Source: CAD feature listing. Evaluate the final solid. Frame: model axes, mm. A direction names the side the tool comes from. Coordinates: 2 decimals unless noted, no trailing zeros. Loops run counter-clockwise (first coordinate to the right, second up) from the corner with the lowest first, then second, coordinate; pieces in that order, holes last. Notation, with made-up numbers: M 34.25,42 L 92.25,42 A16 ccw 92.25,46 Z; hole C 42,62.25 d7. An arc over 180 degrees is marked long. Write each question's results on one line, items separated by ' | '. Start each with the question number.
from build123d import *

# Parameters (mm, degrees)
CHAMFER1_SIZE           = 0.4
EXTRUDE1_START          = -3.25
SKETCH2_R               = 11.925743973
EXTRUDE1_DEPTH          = 3.25
EXTRUDE2_START          = -8.8
SKETCH3_R               = 13.491172398
EXTRUDE2_DEPTH          = 8.8
SKETCH4_W               = 1
SKETCH4_H               = 1.144643989
EXTRUDE3_DEPTH          = 9.5
CUT_EXTRUDE1_DEPTH      = 48.023611133
CUT_EXTRUDE1_DEPTH_BACK = 48.023611133
SKETCH5_R               = 0.520703833
SKETCH6_R               = 1.016043674
CUT_EXTRUDE2_DEPTH      = 0.5
CUT_EXTRUDE3_START      = -0.5
SKETCH7_R               = 1.016043674
CUT_EXTRUDE3_DEPTH      = 0.5


with BuildPart() as part:
    # Sketch1 → Revolve1 (revolve)
    with BuildSketch(Plane.XY, mode=Mode.PRIVATE) as revolve1_sk:
        Polygon((0, 0), (0, 5), (1.5, 5), (1.5, 6.275), (11, 6.275), (11, 8.75), (10.5, 8.75), (10.5, 11), (19.3, 11), (19.3, 6.5), (20.3, 6.5), (20.3, 8.4), (24.65, 8.4), (24.65, 10.75), (27.9, 10.75), (27.9, 3.82), (40, 3.82), (40, 2.3), (38, 2.3), (38, 1.6), (12, 1.6), (12, 0), align=None)
    revolve(revolve1_sk.sketch.rotate(Axis((0, 0, 0), (1, 0, 0)), 90), axis=Axis((0, 0, 0), (1, 0, 0)))

    # Chamfer1
    chamfer1_edges = [part.edges().sort_by_distance(p)[0] for p in [
        (40, 0, -3.82),
    ]]
    chamfer(chamfer1_edges, length=CHAMFER1_SIZE)

    # Sketch2 → Extrude1 (cut)
    with BuildSketch(Plane(origin=(27.9, 0, 0), x_dir=(0, 0, -1), z_dir=(1, 0, 0)).offset(EXTRUDE1_START)):
        Circle(SKETCH2_R)
        Polygon((0, 10.75), (-9.309773091, 5.375), (-9.309773091, -5.375), (0, -10.75), (9.309773091, -5.375), (9.309773091, 5.375), align=None, mode=Mode.SUBTRACT)
    extrude(amount=EXTRUDE1_DEPTH, mode=Mode.SUBTRACT)

    # Sketch3 → Extrude2 (cut)
    with BuildSketch(Plane(origin=(19.3, 0, 0), x_dir=(0, 0, -1), z_dir=(1, 0, 0)).offset(EXTRUDE2_START)):
        Circle(SKETCH3_R)
        Polygon((-5.5, 9.526279442), (-11, 0), (-5.5, -9.526279442), (5.5, -9.526279442), (11, 0), (5.5, 9.526279442), align=None, mode=Mode.SUBTRACT)
    extrude(amount=EXTRUDE2_DEPTH, mode=Mode.SUBTRACT)

    # Sketch4 → Extrude3 (cut)
    with BuildSketch(Plane.ZY.offset(-1.5)):
        with Locations((0, 6.063519509)):
            Rectangle(SKETCH4_W, SKETCH4_H)
    extrude(amount=-EXTRUDE3_DEPTH, mode=Mode.SUBTRACT)

    # Sketch5 → Cut-Extrude1 (cut, two sides: drawn at the far end of the back side and taken through both)
    with BuildSketch(Plane(origin=(0, -4.763139721, 8.25), x_dir=(1, 0, 0), z_dir=(0, -0.5000000000000002, 0.8660254037844386)).offset(-CUT_EXTRUDE1_DEPTH_BACK)):
        with Locations(Location((18.145997854, 9.8, 0), (0, 0, 270))):
            Circle(SKETCH5_R)
    extrude(amount=CUT_EXTRUDE1_DEPTH + CUT_EXTRUDE1_DEPTH_BACK, mode=Mode.SUBTRACT)

    # Sketch6 → Cut-Extrude2 (cut)
    with BuildSketch(Plane(origin=(0, -4.763139721, 8.25), x_dir=(1, 0, 0), z_dir=(0, -0.5000000000000002, 0.8660254037844386))):
        with Locations(Location((16.808700708, 2.994097786, 0), (0, 0, 270))):
            Circle(SKETCH6_R)
    extrude(amount=-CUT_EXTRUDE2_DEPTH, mode=Mode.SUBTRACT)

    # Sketch7 → Cut-Extrude3 (cut)
    with BuildSketch(Plane(origin=(0, 4.763139721, -8.25), x_dir=(-1, 0, 0), z_dir=(0, 0.49999999999999944, -0.8660254037844389)).offset(CUT_EXTRUDE3_START)):
        with Locations(Location((-16.808700708, 2.994097786, 0), (0, 0, 270))):
            Circle(SKETCH7_R)
    extrude(amount=CUT_EXTRUDE3_DEPTH, mode=Mode.SUBTRACT)


solid = part.part
Item 1: Cut plane A-A (x = 3). Output: boundary loops of the cut face in (y, z) (3 decimals).
Item 2: First-contact query: pin 1 Ø2 at (x, z) = (11.5, 5) entering from -Y; pin 2 Ø0.8 at (x, y) = (4, 6) entering from +Z; pin 3 Ø6 at (x, z) = (4.5, -8) entering from -Y. Flat tips, straight axial feed; report the tip coordinate or a pass-through.
Item 3: Line query: probe 1 along Y at (x, z) = (10.8, 0) (3 decimals); probe 2 along X at (y, z) = (4.25, -5); probe 3 along Y at (x, z) = (17.75, 0). Output: solid intervals per line, ascending.
Item 4: Mould query, pull axis Z, two halves, no side actions, for faces 1 (the flat face through (19.3, -6.5, 2.3)), 2 (the flat face through (38, 0, -2)), 3 (the cylindrical face through (22.505, -2.523, 8.012)). Classes: +Z half, -Z half, draft (parallel to the pull), parting line (faces both ways), or undercut.
Item 5: Access query for faces 4 (the flat face through (15, 9.526, 0)), 5 (the flat face through (26.252, -8.025, 4.72)), 6 (the flat face through (26.25, 8.1, 4.59)). Directions: +Z, -Z, +X, -X, +Y, -Y. A direction counts if a zero-diameter tool reaches every point of the face in a straight line with its end or side. Return the directions, or none.
Response values:
1) outline: M 5.491,-0.5 L 5.491,0.5 L 6.255,0.5 A6.275 ccw long 6.255,-0.5 Z
2) pin 1: stops at y = -9.53 | pin 2: stops at z = 2.83 | pin 3: stops at y = -3.79
3) probe 1: y = -9.526 to -8.75, -6.275 to 5.491, 8.75 to 9.526 | probe 2: x = 11 to 19.3, 20.3 to 27.9 | probe 3: y = -9.53 to -1.6, 1.6 to 9.53
4) face 1: draft | face 2: undercut | face 3: parting line
5) face 4: +Z, -Z, -X, +Y | face 5: +Z, +X, -Y | face 6: +Z, +X, +Y
